Can you work these out from the model? Positions are in its coordinate system, mm. Coordinates: 2 decimals unless noted, no trailing zeros. Answer as a JSON object with one key per item and string values.
from build123d import *

# Parameters (mm, degrees)
SKETCH_1_W             = 800
SKETCH_1_H             = 5
EXTRUDE_1_DEPTH        = 0.5
SKETCH_2_W             = 5
SKETCH_2_H             = 5
EXTRUDE_2_DEPTH        = 1.7
PATTERN_LINEAR_1_COUNT = 48
PATTERN_LINEAR_1_PITCH = 16.666666667


with BuildPart() as part:
    # 草图1 → 凸台-拉伸1 (new body)
    with BuildSketch(Plane(origin=(0, 0, 0), x_dir=(1, 0, 0), z_dir=(0, 1, 0))):
        Rectangle(SKETCH_1_W, SKETCH_1_H)
    extrude(amount=EXTRUDE_1_DEPTH)

    # 草图2 → 凸台-拉伸2 (add)
    with BuildSketch(Plane(origin=(0, 0.5, 0), x_dir=(1, 0, 0), z_dir=(0, 1, 0))):
        with Locations((-397.5, 0)):
            Rectangle(SKETCH_2_W, SKETCH_2_H)
    extrude_2 = extrude(amount=EXTRUDE_2_DEPTH)

    # 阵列(线性)1: 凸台-拉伸2 ×48
    with Locations(*[(i * PATTERN_LINEAR_1_PITCH, 0, 0) for i in range(1, PATTERN_LINEAR_1_COUNT)]):
        add(extrude_2)


solid = part.part
Item 1: I want a section at A-A, the plane y = 1.55. Give the number of separate pieces and of enclosed holes in the cut face, plus the area to 3 significant figures.
Answers follow:
{"separate pieces": "48", "enclosed holes": "0", "area": "1,200 mm^2"}
Item 2: Please list where this line runs through material, in increasing order: line 1 (Y direction, x = -327, z = -0.1).
Answers follow:
{"line 1": "y = 0 to 0.5"}
Item 3: I'm going to push flat-ended pins straight in: pin 1 (0.5 mm diameter, centred on y = 1.5, z = 1, fed in from +X); pin 2 (2.5 mm diameter, centred on x = -3, z = 1, fed in from +Y). Where does each tip first touch, or does it pass through?
Answers follow:
{"pin 1": "stops at x = 388.33", "pin 2": "stops at y = 0.5"}
